Geometry check sheet. Reference: drawing and pictorial views, mm from the part's lowest x, y, z. A direction names the side the tool comes from. Round coordinates to 2 decimals unless told otherwise and drop trailing zeros. Order: outer loops, then holes, each group sorted by start corner. A loop starts at its lowest first (then second) coordinate and runs counter-clockwise, first axis right, second up.
(1) Sectioned sample at D-D (x = 7). Record the boundary of the cut face in (y, z) (1 decimal), plus the area to 3 significant figures.
(2) Sectioned sample at B-B (y = 86). Record the boundary of the cut face in (x, z) (1 decimal), plus the area to 4 significant figures.
(3) Go/stop test with flat-tipped pins: pin 1 (8 mm diameter, centred on x = 69.85, z = 19.05, fed in from -Y); pin 2 (17.5 mm diameter, centred on x = 45.5, y = 80, fed in from -Z) (3 decimals); pin 3 (1 mm diameter, centred on x = 33, z = 7.5, fed in from +Y) (3 decimals); pin 4 (3 mm diameter, centred on x = 81.6, y = 15.49, fed in from -Z). Record where each tip stops, or that it passes through.
(4) Set-up check for the marked faces 1, 2 and 3: record each of +Z, -Z, +X, -X, +Y, -Y from which the full face is reachable in a straight line by a thin tool's end or side.
(5) Material ranges on line 1 along X through (y, z) = (35, 19); line 2 along Z through (x, y) = (31.75, 36.75); line 3 along X through (y, z) = (67.5, 9) (1 decimal), recorded low to high.
(6) Sectioned sample at A-A (x = 31.75). Record the boundary of the cut face in (y, z) (1 decimal), plus the area to 3 significant figures.
(7) Sectioned sample at C-C (z = 19.05). Record the boundary of the cut face in (x, y) (1 decimal).
(8) Release check for a two-part mould opening along X. For the marked faces 4, 5 and 6 record: +X half, -X half, draft (parallel to the pull), parting line (faces both ways), or undercut.
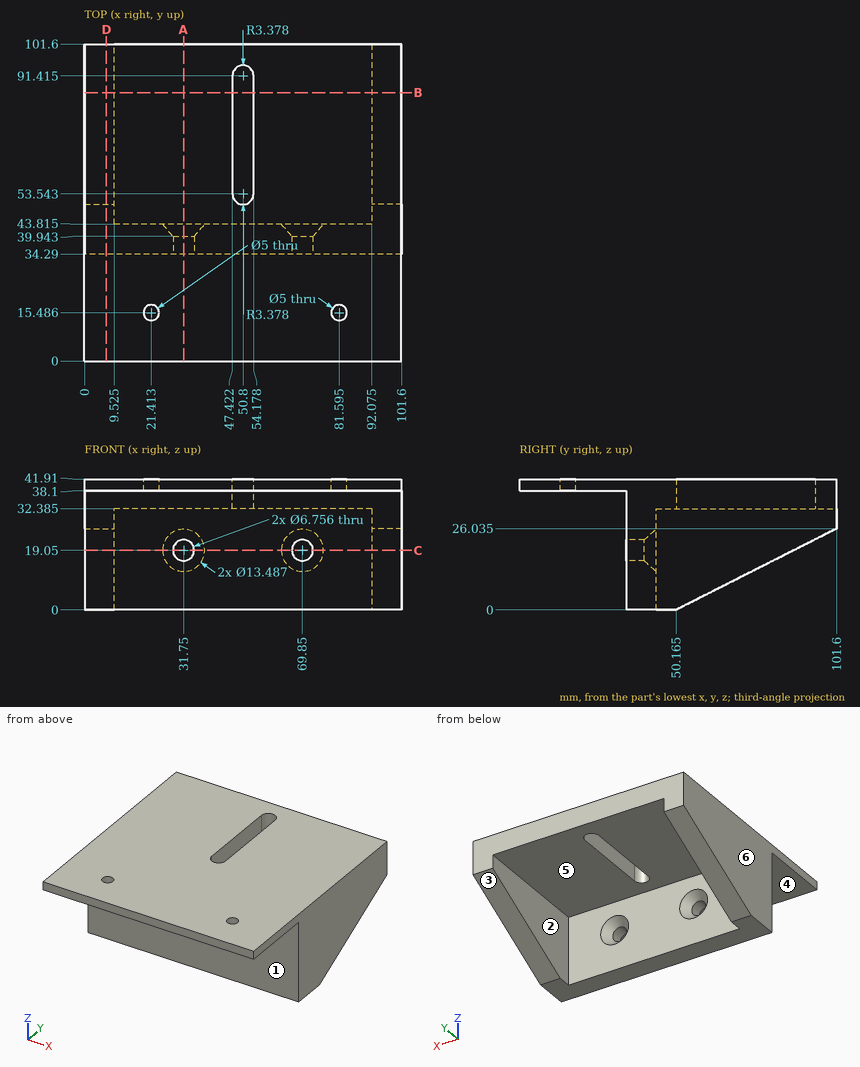
Answer below:
1. outline: (0, 38.1) - (34.3, 38.1) - (34.3, 0) - (50.2, 0) - (101.6, 26) - (101.6, 41.9) - (0, 41.9) - close
1. area: 2,280 mm2
2. outline: (0, 18.1) - (9.5, 18.1) - (9.5, 32.4) - (47.4, 32.4) - (47.4, 41.9) - (0, 41.9) - close; (54.2, 32.4) - (92.1, 32.4) - (92.1, 18.1) - (101.6, 18.1) - (101.6, 41.9) - (54.2, 41.9) - close
2. area: 1,175 mm2
3. pin 1: stops at y = 34.29
3. pin 2: stops at z = 32.385
3. pin 3: stops at y = 43.815
3. pin 4: passes through
4. face 1: -Z, +X, -X, -Y
4. face 2: -Z, +Y
4. face 3: -Z, +X, -X, +Y
5. line 1: x = 0 to 28.37, 35.13 to 66.47, 73.23 to 101.6
5. line 2: z = 0 to 15.67, 22.43 to 41.91
5. line 3: x = 0 to 9.5, 92.1 to 101.6
6. outline: (0, 38.1) - (34.3, 38.1) - (34.3, 22.4) - (39.9, 22.4) - (43.8, 25.8) - (43.8, 32.4) - (101.6, 32.4) - (101.6, 41.9) - (0, 41.9) - close; (34.3, 0) - (43.8, 0) - (43.8, 12.3) - (39.9, 15.7) - (34.3, 15.7) - close
6. area: 1,000 mm2
7. outline: (0, 34.3) - (28.4, 34.3) - (28.4, 39.9) - (25, 43.8) - (9.5, 43.8) - (9.5, 87.8) - (0, 87.8) - close; (35.1, 34.3) - (66.5, 34.3) - (66.5, 39.9) - (63.1, 43.8) - (38.5, 43.8) - (35.1, 39.9) - close; (73.2, 34.3) - (101.6, 34.3) - (101.6, 87.8) - (92.1, 87.8) - (92.1, 43.8) - (76.6, 43.8) - (73.2, 39.9) - close
8. face 4: draft
8. face 5: undercut
8. face 6: -X half
